```python
from build123d import *

# Parameters (mm, degrees)
ESQUISSE1_W              = 40
ESQUISSE1_H              = 40
BOSS_EXTRU_1_DEPTH       = 50
ESQUISSE2_R              = 5
ENL_V_MAT_EXTRU_1_DEPTH  = 41
ESQUISSE3_R              = 5
ENL_V_MAT_EXTRU_2_DEPTH  = 41
ESQUISSE4_W              = 22
ESQUISSE4_H              = 14
ENL_V_MAT_EXTRU_3_DEPTH  = 29
ESQUISSE5_W              = 14
ESQUISSE5_H              = 20
ENL_V_MAT_EXTRU_4_DEPTH  = 29
ESQUISSE6_W              = 20
ESQUISSE6_H              = 14
ENL_V_MAT_EXTRU_5_DEPTH  = 24
ESQUISSE7_W              = 14
ESQUISSE7_H              = 22
ENL_V_MAT_EXTRU_6_DEPTH  = 24
ESQUISSE10_R             = 11.25
ENL_V_MAT_EXTRU_9_DEPTH  = 7
ESQUISSE11_R             = 12.75
ENL_V_MAT_EXTRU_10_DEPTH = 1.5
ESQUISSE14_R             = 11.25
ENL_V_MAT_EXTRU_11_DEPTH = 7
ESQUISSE15_R             = 12.75
ENL_V_MAT_EXTRU_12_DEPTH = 1.5
ESQUISSE16_W             = 40
ESQUISSE16_H             = 40
BOSS_EXTRU_2_DEPTH       = 7
ESQUISSE17_R             = 2.25
ENL_V_MAT_EXTRU_13_DEPTH = 15
ESQUISSE18_W             = 7
ESQUISSE18_H             = 3
ENL_V_MAT_EXTRU_14_DEPTH = 12
ESQUISSE19_W             = 3.5
ESQUISSE19_H             = 7.5
ENL_V_MAT_EXTRU_15_DEPTH = 12


with BuildPart() as part:
    # Esquisse1 → Boss.-Extru.1 (new body)
    with BuildSketch(Plane.XY):
        with Locations((-20, 20)):
            Rectangle(ESQUISSE1_W, ESQUISSE1_H)
    extrude(amount=BOSS_EXTRU_1_DEPTH)

    # Esquisse2 → Enlèv. mat.-Extru.1 (cut, through all)
    with BuildSketch(Plane(origin=(0, 40, 0), x_dir=(1, 0, 0), z_dir=(0, 1, 0))):
        with Locations(Location((-20, -15, 0), (0, 0, 270))):  # turned: the seam where the file's is
            Circle(ESQUISSE2_R)
    extrude(amount=-ENL_V_MAT_EXTRU_1_DEPTH, mode=Mode.SUBTRACT)

    # Esquisse3 → Enlèv. mat.-Extru.2 (cut, through all)
    with BuildSketch(Plane.ZY.offset(40)):
        with Locations((35, 20)):
            Circle(ESQUISSE3_R)
    extrude(amount=-ENL_V_MAT_EXTRU_2_DEPTH, mode=Mode.SUBTRACT)

    # Esquisse4 → Enlèv. mat.-Extru.3 (cut)
    with BuildSketch(Plane.ZY.offset(40)):
        with Locations((11, 20)):
            Rectangle(ESQUISSE4_W, ESQUISSE4_H)
    extrude(amount=-ENL_V_MAT_EXTRU_3_DEPTH, mode=Mode.SUBTRACT)

    # Esquisse5 → Enlèv. mat.-Extru.4 (cut)
    with BuildSketch(Plane.XZ):
        with Locations((-20, 35)):
            Rectangle(ESQUISSE5_W, ESQUISSE5_H)
    extrude(amount=-ENL_V_MAT_EXTRU_4_DEPTH, mode=Mode.SUBTRACT)

    # Esquisse6 → Enlèv. mat.-Extru.5 (cut)
    with BuildSketch(Plane(origin=(0, 0, 0), x_dir=(0, 0, -1), z_dir=(1, 0, 0))):
        with Locations((-15, 20)):
            Rectangle(ESQUISSE6_W, ESQUISSE6_H)
    extrude(amount=-ENL_V_MAT_EXTRU_5_DEPTH, mode=Mode.SUBTRACT)

    # Esquisse7 → Enlèv. mat.-Extru.6 (cut)
    with BuildSketch(Plane(origin=(0, 40, 0), x_dir=(1, 0, 0), z_dir=(0, 1, 0))):
        with Locations((-20, -39)):
            Rectangle(ESQUISSE7_W, ESQUISSE7_H)
    extrude(amount=-ENL_V_MAT_EXTRU_6_DEPTH, mode=Mode.SUBTRACT)

    # Esquisse10 → Enlèv. mat.-Extru.9 (cut)
    with BuildSketch(Plane(origin=(0, 40, 0), x_dir=(1, 0, 0), z_dir=(0, 1, 0))):
        with Locations(Location((-20, -15, 0), (0, 0, 270))):  # turned: the seam where the file's is
            Circle(ESQUISSE10_R)
    extrude(amount=-ENL_V_MAT_EXTRU_9_DEPTH, mode=Mode.SUBTRACT)

    # Esquisse11 → Enlèv. mat.-Extru.10 (cut)
    with BuildSketch(Plane(origin=(0, 40, 0), x_dir=(1, 0, 0), z_dir=(0, 1, 0))):
        with Locations(Location((-20, -15, 0), (0, 0, 270))):  # turned: the seam where the file's is
            Circle(ESQUISSE11_R)
    extrude(amount=-ENL_V_MAT_EXTRU_10_DEPTH, mode=Mode.SUBTRACT)

    # Esquisse14 → Enlèv. mat.-Extru.11 (cut)
    with BuildSketch(Plane.ZY.offset(40)):
        with Locations((35, 20)):
            Circle(ESQUISSE14_R)
    extrude(amount=-ENL_V_MAT_EXTRU_11_DEPTH, mode=Mode.SUBTRACT)

    # Esquisse15 → Enlèv. mat.-Extru.12 (cut)
    with BuildSketch(Plane.ZY.offset(40)):
        with Locations((35, 20)):
            Circle(ESQUISSE15_R)
    extrude(amount=-ENL_V_MAT_EXTRU_12_DEPTH, mode=Mode.SUBTRACT)

    # Esquisse16 → Boss.-Extru.2 (add)
    with BuildSketch(Plane.XY.offset(50)):
        with Locations((-20, 20)):
            Rectangle(ESQUISSE16_W, ESQUISSE16_H)
    extrude(amount=BOSS_EXTRU_2_DEPTH)

    # Esquisse17 → Enlèv. mat.-Extru.13 (cut)
    with BuildSketch(Plane.XY.offset(57)):
        with Locations((-30, 7.5)):
            Circle(ESQUISSE17_R)
        with Locations((-7.5, 30)):
            Circle(ESQUISSE17_R)
    extrude(amount=-ENL_V_MAT_EXTRU_13_DEPTH, mode=Mode.SUBTRACT)

    # Esquisse18 → Enlèv. mat.-Extru.14 (cut)
    with BuildSketch(Plane.XZ):
        with Locations((-30, 51.5)):
            Rectangle(ESQUISSE18_W, ESQUISSE18_H)
    extrude(amount=-ENL_V_MAT_EXTRU_14_DEPTH, mode=Mode.SUBTRACT)

    # Esquisse19 → Enlèv. mat.-Extru.15 (cut)
    with BuildSketch(Plane(origin=(0, 0, 0), x_dir=(0, 0, -1), z_dir=(1, 0, 0))):
        with Locations((-51.25, 30)):
            Rectangle(ESQUISSE19_W, ESQUISSE19_H)
    extrude(amount=-ENL_V_MAT_EXTRU_15_DEPTH, mode=Mode.SUBTRACT)


solid = part.part
```
Input: part model. Units: mm. Frame: model coordinates. A direction names the side the tool comes from. Round coordinates to 2 decimals unless told otherwise and drop trailing zeros. Write each loop counter-clockwise with the first axis right and the second up, starting at its lowest first coordinate (ties: lowest second). Pieces come first, ordered by that corner, then holes. Notation, with made-up numbers: M 87.5,24.5 L 146.5,24.5 A16 ccw 146.5,40.5 Z; hole C 29.5,48 d9. An arc over 180 degrees is marked long. Write each question's results on one line, items separated by ' | '.
Q1. Line query: line 1 along X through (y, z) = (22, 26); line 2 along X through (y, z) = (36, 15); line 3 along Y through (x, z) = (-37.5, 4.5). Output: solid intervals per line, ascending.
Results:
line 1: x = -33 to -27, -13 to 0 | line 2: x = -40 to -31.25, -8.75 to 0 | line 3: y = 0 to 13, 27 to 40
Q2. Draft query along X for faces 1 (the face through (-12, 30, 51)), 2 (the face through (-33.5, 6, 51)), 3 (the face through (-11, 20, 2)), 4 (the face through (-6, 26.25, 51)). Return one class per face: released by +X, released by -X, zero draft, split by the parting line, or undercut.
Results:
face 1: released by +X | face 2: undercut | face 3: released by -X | face 4: zero draft
Q3. Pin query (flat end, axial travel): P1, Ø6, axis at y = 21.5, z = 37.5, coming from the -X side; P2, Ø0.9, axis at x = -28.5, z = 51, coming from the -Y side; P3, Ø1.5, axis at x = -20, z = 46.5, coming from the +Y side. Return the tip coordinate at first contact, or that it passes through.
Results:
P1: stops at x = -33 | P2: stops at y = 12 | P3: stops at y = 16
Q4. Section query A-A (x = -37). Return loops of the section in (y, z), and give its area (3 significant figures).
Results:
outline: M 0,0 L 13,0 L 13,22 L 27,22 L 27,0 L 40,0 L 40,57 L 0,57 Z; hole C 20,35 d22.5 | area: 1,570 mm^2
Q5. Access query for faces 5 (the face through (-5, 30, 53)), 6 (the face through (-30, 5, 53)), 7 (the face through (-9.748, 30.099, 45.802)), 8 (the face through (-20, 16, 47)), 9 (the face through (-7, 17, 31)). Directions: +Z, -Z, +X, -X, +Y, -Y. A direction counts if a zero-diameter tool reaches every point of the face in a straight line with its end or side. Return the directions, or none.
Results:
face 5: +X | face 6: -Y | face 7: +Z | face 8: +Y | face 9: +X, -X
Q6. Section query B-B (z = 15). Return loops of the section in (x, y), and give its area (3 significant figures).
Results:
outline: M -40,0 L -25,0 L -25,13 L -40,13 Z; M -40,27 L -25,27 L -25,33 L -31.25,33 L -31.25,38.5 L -32.75,38.5 L -32.75,40 L -40,40 Z; M -15,0 L 0,0 L 0,13 L -15,13 Z; M -15,27 L 0,27 L 0,40 L -7.25,40 L -7.25,38.5 L -8.75,38.5 L -8.75,33 L -15,33 Z | area: 688 mm^2
Q7. Section query C-C (y = 17.5). State how many separate pieces and enclosed holes the cut face has, and give its area (3 significant figures).
Results:
separate pieces: 4 | enclosed holes: 0 | area: 710 mm^2
